Design review of the part built by this model. Coordinates are the model's own, in mm. Face numbers are marked on the shaded views. Coordinates: 2 decimals unless noted, no trailing zeros. Write each loop counter-clockwise with the first axis right and the second up, starting at its lowest first coordinate (ties: lowest second). Pieces come first, ordered by that corner, then holes.
Q1. The part is to be moulded in two halves that separate along X. For the marked faces 1, 2 and 3, say which applies: released by +X, released by -X, zero draft, split by the parting line, or undercut.
Q2. Take a section at A-A, the plane z = 59.15. Write out the cut boundary in (x, y), plus the area to 3 significant figures.
Q3. Take a section at D-D, the plane y = -143. Write out the cut boundary in (x, z).
Q4. Take a section at C-C, the plane z = 15.5. Write out the cut boundary in (x, y), plus the area to 3 significant figures.
Q5. Take a section at B-B, the plane x = 17.4. Write out the cut boundary in (y, z).
Q6. For pin 1 Ø1 at (y, z) = (-142.5, 28.5) entering from -X; pin 2 Ø3 at (y, z) = (-148.5, 21) entering from -X; pin 3 Ø7.5 at (x, y) = (17.4, -148.62) entering from -Z, all flat-tipped, find the tip position at first contact; note any pin that passes through.
Q7. For L1, parallel to X at y = -148.5, z = 19; L2, parallel to X at y = -152, z = 28.5; L3, parallel to X at y = -150.25, z = 58.5, list the stretches that pass through material, from the lowest coordinate up.
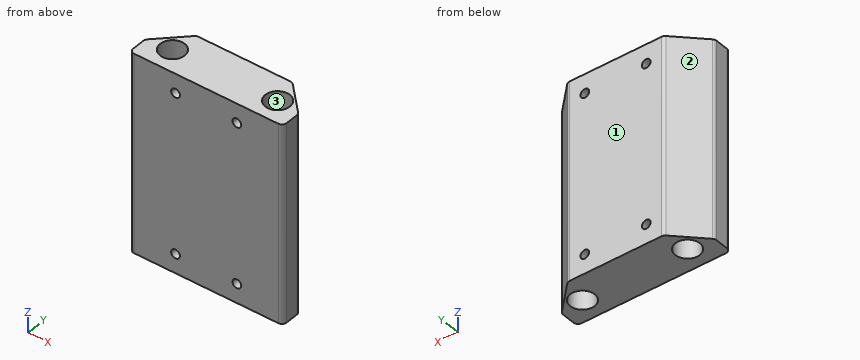
from build123d import *

# Parameters (mm, degrees)
SKETCH1_W           = 50.8
SKETCH1_H           = 16
SKETCH1_R           = 4.05
BOSS_EXTRUDE1_DEPTH = 65.5
FILLET1_R           = 1.5
CHAMFER1_SIZE       = 9.525
FILLET2_R           = 1.5
SKETCH3_R           = 1.45
CUT_EXTRUDE1_DEPTH  = 17


with BuildPart() as part:
    # Sketch1 → Boss-Extrude1 (new body)
    with BuildSketch(Plane.XY):
        with Locations((-0.262087977, -148.149956673)):
            Rectangle(SKETCH1_W, SKETCH1_H)
        with Locations((-17.4, -148.618426491)):
            Circle(SKETCH1_R, mode=Mode.SUBTRACT)
        with Locations((17.4, -148.618426491)):
            Circle(SKETCH1_R, mode=Mode.SUBTRACT)
    extrude(amount=BOSS_EXTRUDE1_DEPTH)

    # Fillet1
    fillet1_edges = [part.edges().sort_by_distance(p)[0] for p in [
        (25.137912023, -156.149956673, 32.75),
        (-25.662087977, -156.149956673, 32.75),
    ]]
    fillet(fillet1_edges, radius=FILLET1_R)

    # Chamfer1
    chamfer1_edges = [part.edges().sort_by_distance(p)[0] for p in [
        (-25.662087977, -140.149956673, 32.75),
        (25.137912023, -140.149956673, 32.75),
    ]]
    chamfer(chamfer1_edges, length=CHAMFER1_SIZE)

    # Fillet2
    fillet2_edges = [part.edges().sort_by_distance(p)[0] for p in [
        (-16.137087977, -140.149956673, 32.75),
        (15.612912023, -140.149956673, 32.75),
        (25.137912023, -149.674956673, 32.75),
        (-25.662087977, -149.674956673, 32.75),
    ]]
    fillet(fillet2_edges, radius=FILLET2_R)

    # Sketch3 → Cut-Extrude1 (cut, through all)
    with BuildSketch(Plane.XZ.offset(156.149956673)):
        with Locations((-10.422087977, 59.15)):
            Circle(SKETCH3_R)
        with Locations((9.897912023, 59.15)):
            Circle(SKETCH3_R)
        with Locations((-10.422087977, 6.35)):
            Circle(SKETCH3_R)
        with Locations((9.897912023, 6.35)):
            Circle(SKETCH3_R)
    extrude(amount=-CUT_EXTRUDE1_DEPTH, mode=Mode.SUBTRACT)


solid = part.part
Responses:
1. face 1: zero draft
1. face 2: released by -X
1. face 3: undercut
2. outline: (-25.66, -154.65) arc R1.5 ccw to (-24.16, -156.15) - (-11.87, -156.15) - (-11.87, -140.15) - (-15.52, -140.15) arc R1.5 ccw to (-16.58, -140.59) - (-25.22, -149.24) arc R1.5 ccw to (-25.66, -150.3) - close; (-8.97, -156.15) - (8.45, -156.15) - (8.45, -140.15) - (-8.97, -140.15) - close; (11.35, -156.15) - (23.64, -156.15) arc R1.5 ccw to (25.14, -154.65) - (25.14, -150.3) arc R1.5 ccw to (24.7, -149.24) - (16.05, -140.59) arc R1.5 ccw to (14.99, -140.15) - (11.35, -140.15) - close; hole circle Ø8.1 at (-17.4, -148.62); hole circle Ø8.1 at (17.4, -148.62)
2. area: 525 mm2
3. outline: (-18.99, 0) - (18.46, 0) - (18.46, 65.5) - (-18.99, 65.5) - close; hole circle Ø2.9 at (-10.42, 6.35); hole circle Ø2.9 at (-10.42, 59.15); hole circle Ø2.9 at (9.9, 6.35); hole circle Ø2.9 at (9.9, 59.15)
4. outline: (-25.66, -154.65) arc R1.5 ccw to (-24.16, -156.15) - (23.64, -156.15) arc R1.5 ccw to (25.14, -154.65) - (25.14, -150.3) arc R1.5 ccw to (24.7, -149.24) - (16.05, -140.59) arc R1.5 ccw to (14.99, -140.15) - (-15.52, -140.15) arc R1.5 ccw to (-16.58, -140.59) - (-25.22, -149.24) arc R1.5 ccw to (-25.66, -150.3) - close; hole circle Ø8.1 at (-17.4, -148.62); hole circle Ø8.1 at (17.4, -148.62)
4. area: 618 mm2
5. outline: (-156.15, 0) - (-152.67, 0) - (-152.67, 65.5) - (-156.15, 65.5) - close; (-144.57, 0) - (-141.94, 0) - (-141.94, 65.5) - (-144.57, 65.5) - close
6. pin 1: stops at x = -18.99
6. pin 2: stops at x = -25.63
6. pin 3: passes through
7. L1: x = -24.49 to -21.45, -13.35 to 13.35, 21.45 to 23.96
7. L2: x = -25.66 to -19.63, -15.17 to 15.17, 19.63 to 25.14
7. L3: x = -25.66 to -21.11, -13.69 to -11.72, -9.13 to 8.6, 11.19 to 13.69, 21.11 to 25.14
